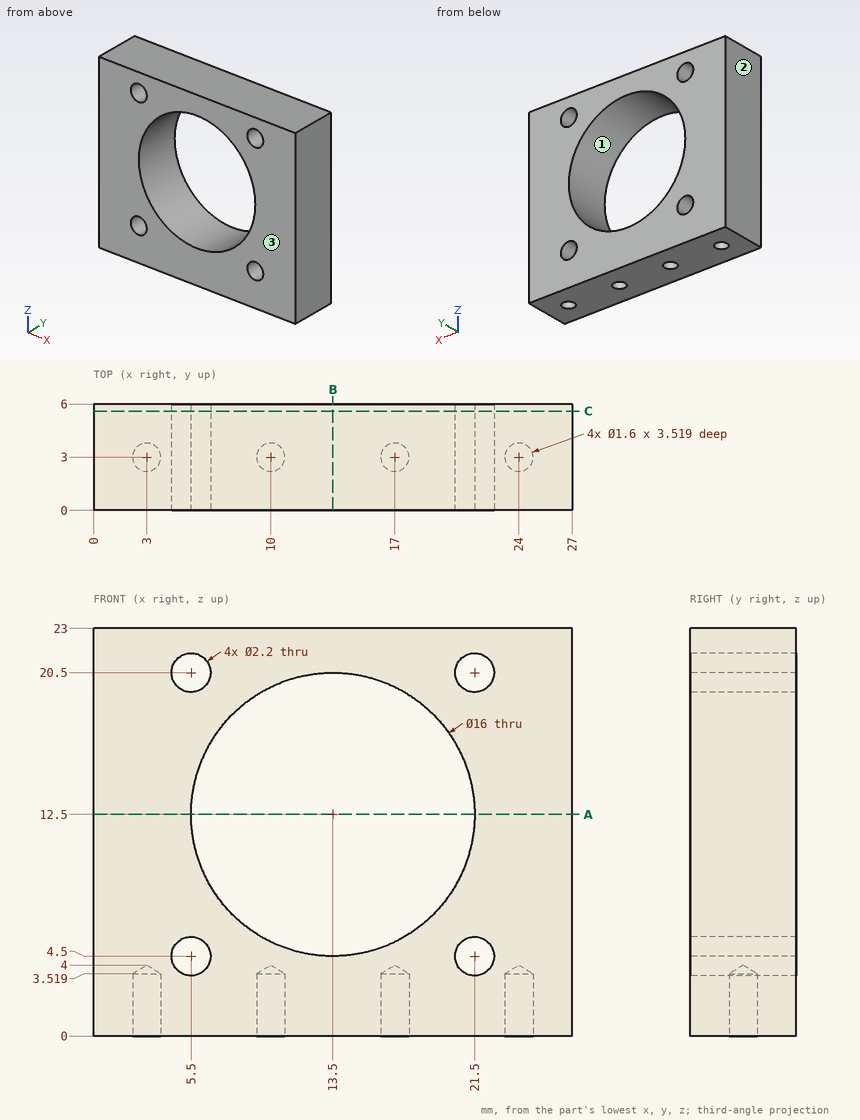
Here's the drawing with two shaded views (mm, measured from the low corner). I have some questions. Coordinates: 2 decimals unless noted, no trailing zeros. Loops run counter-clockwise (first coordinate to the right, second up) from the corner with the lowest first, then second, coordinate; pieces in that order, holes last. Notation, with made-up numbers: (-15, 34.5) -> (40, 34.5) arc R9 cw to (40, 38.5) -> close; hole circle Ø4 at (3.25, 35). An arc over 180 degrees is marked (long way). Put each result on its own line as item: value. Start each with the question number.
Q1. Thinking about a two-plate mould opening in X: for the marked faces 1, 2 and 3, which applies, pulls with the +X half, pulls with the -X half, needs draft (parallel to the pull), parting line crosses it, or undercut?
Q2. I want a section at A-A (z = 12.5). Write out the boundary of the cut face in (x, y).
Q3. I want a section at C-C (y = 5.6). Write out the boundary of the cut face in (x, z).
Q4. I want a section at B-B (x = 13.5). Write out the boundary of the cut face in (y, z).
Q5. If I drill on line 1 (X direction, y = 3, z = 2.85); line 2 (Y direction, x = 24, z = 2.85); line 3 (Z direction, x = 13.5, y = 2.75), over which ranges is the centre line in solid material (lowest first)? Write a range as [from, to].
Q6. I'm going to push flat-ended pins straight in: P1, Ø1.3, axis at x = 24, y = 3, coming from the -Z side; P2, Ø0.8, axis at x = 3, y = 3, coming from the -Z side. Where does each tip first touch, or does it pass through?
Taken from the geometry:
1. face 1: undercut
1. face 2: pulls with the -X half
1. face 3: needs draft
2. outline: (0, 0) -> (5.5, 0) -> (5.5, 6) -> (0, 6) -> close; (21.5, 0) -> (27, 0) -> (27, 6) -> (21.5, 6) -> close
3. outline: (0, 0) -> (27, 0) -> (27, 23) -> (0, 23) -> close; hole circle Ø2.2 at (5.5, 4.5); hole circle Ø2.2 at (5.5, 20.5); hole circle Ø16 at (13.5, 12.5); hole circle Ø2.2 at (21.5, 4.5); hole circle Ø2.2 at (21.5, 20.5)
4. outline: (0, 0) -> (6, 0) -> (6, 4.5) -> (0, 4.5) -> close; (0, 20.5) -> (6, 20.5) -> (6, 23) -> (0, 23) -> close
5. line 1: x = [0, 2.2], [3.8, 9.2], [10.8, 16.2], [17.8, 23.2], [24.8, 27]
5. line 2: y = [0, 2.2], [3.8, 6]
5. line 3: z = [0, 4.5], [20.5, 23]
6. P1: stops at z = 3.61
6. P2: stops at z = 3.76
